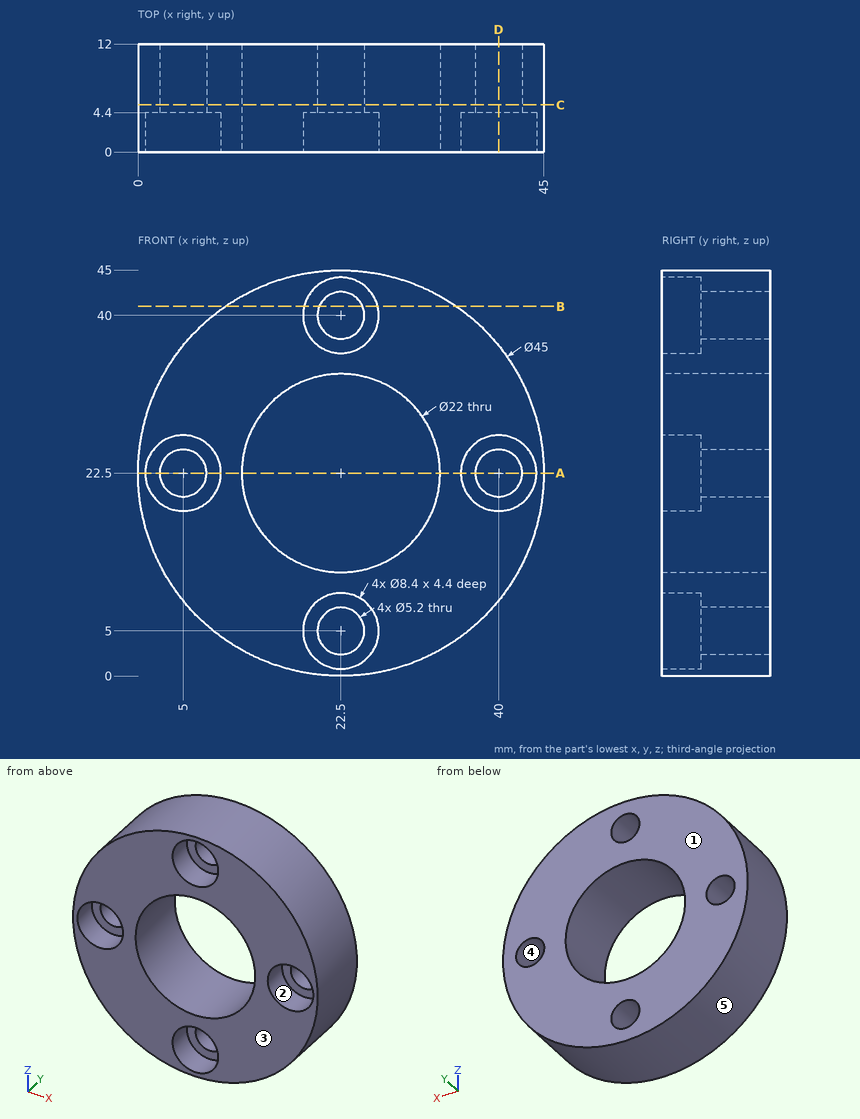
Part print with two shaded views. Sizes in mm from the minimum x, y, z corner. A direction names the side the tool comes from. Round coordinates to 2 decimals unless told otherwise and drop trailing zeros. Loops run counter-clockwise (first coordinate to the right, second up) from the corner with the lowest first, then second, coordinate; pieces in that order, holes last.
Item 1: Saw through at A-A (z = 22.5). List the corners of the cut face in (x, y), then the cut area to 3 significant figures.
Item 2: Saw through at C-C (y = 5.25). List the corners of the cut face in (x, z).
Item 3: Two-plate mould, pull along Z, no slides. Class the marked faces 3, 4 and 5: released by +Z, released by -Z, zero draft, split by the parting line, or undercut.
Item 4: Saw through at D-D (x = 40). List the corners of the cut face in (y, z).
Item 5: Which spindle directions (+Z, -Z, +X, -X, +Y, -Y) get a long thin tool onto all of the face, cutting with end or side? Do the marked faces 1 and 2. Say none if no direction does.
Item 6: Pin check, flat tips, straight feed: P1, Ø1.5, axis at x = 5.5, y = 4, coming from the -Z side; P2, Ø3, axis at y = 2.5, z = 20.5, coming from the -X side; P3, Ø4, axis at y = 3.5, z = 14, coming from the -X side. Stop position of each tip, or through.
Item 7: Saw through at B-B (z = 41). List the corners of the cut face in (x, y).
Item 8: Drill centre lines: line 1 along X through (y, z) = (5.5, 22.5); line 2 along X through (y, z) = (3.35, 22.5); line 3 along Z through (x, y) = (22, 8.25). Where is each one in solid material? Low to high.
Worked answers:
1. outline: (0, 0) - (0.8, 0) - (0.8, 4.4) - (2.4, 4.4) - (2.4, 12) - (0, 12) - close; (7.6, 4.4) - (9.2, 4.4) - (9.2, 0) - (11.5, 0) - (11.5, 12) - (7.6, 12) - close; (33.5, 0) - (35.8, 0) - (35.8, 4.4) - (37.4, 4.4) - (37.4, 12) - (33.5, 12) - close; (42.6, 4.4) - (44.2, 4.4) - (44.2, 0) - (45, 0) - (45, 12) - (42.6, 12) - close
1. area: 123 mm2
2. outline: circle Ø45 at (22.5, 22.5); hole circle Ø5.2 at (5, 22.5); hole circle Ø22 at (22.5, 22.5); hole circle Ø5.2 at (22.5, 5); hole circle Ø5.2 at (22.5, 40); hole circle Ø5.2 at (40, 22.5)
3. face 3: zero draft
3. face 4: undercut
3. face 5: split by the parting line
4. outline: (0, 8.36) - (12, 8.36) - (12, 19.9) - (4.4, 19.9) - (4.4, 18.3) - (0, 18.3) - close; (0, 26.7) - (4.4, 26.7) - (4.4, 25.1) - (12, 25.1) - (12, 36.64) - (0, 36.64) - close
5. face 1: +Z, -Z, +X, -X, +Y
5. face 2: -Y
6. P1: stops at z = 6.94
6. P2: stops at x = 0.01
6. P3: stops at x = 0.96
7. outline: (9.69, 0) - (18.42, 0) - (18.42, 4.4) - (20.1, 4.4) - (20.1, 12) - (9.69, 12) - close; (24.9, 4.4) - (26.58, 4.4) - (26.58, 0) - (35.31, 0) - (35.31, 12) - (24.9, 12) - close
8. line 1: x = 0 to 2.4, 7.6 to 11.5, 33.5 to 37.4, 42.6 to 45
8. line 2: x = 0 to 0.8, 9.2 to 11.5, 33.5 to 35.8, 44.2 to 45
8. line 3: z = 0.01 to 2.45, 7.55 to 11.51, 33.49 to 37.45, 42.55 to 44.99
